Verification items for the finished model (mm, model axes). Face numbers are marked on the shaded views. A direction names the side the tool comes from. Coordinates: 2 decimals unless noted, no trailing zeros. Order: outer loops, then holes, each group sorted by start corner. A loop starts at its lowest first (then second) coordinate and runs counter-clockwise, first axis right, second up. Notation, with made-up numbers: M -13.75,-20.5 L 32.25,-20.5 A20 ccw 32.25,-12.5 Z; hole C -23,75.5 d1. An arc over 180 degrees is marked long. Answer as a JSON object with one key per item and string values. Group by question number.
(1) Cross-section at A-A (x = -34.25). Enter the section's corners in (y, z), plus the area to 3 significant figures.
(2) Cross-section at C-C (z = 10.25). Enter the section's corners in (x, y).
(3) Cross-section at B-B (y = -96). Enter the section's corners in (x, z), plus the area to 3 significant figures.
(4) Cross-section at D-D (x = -40.75). Enter the section's corners in (y, z).
(5) Gauge pin test, flat ends, axial feed: pin 1 Ø1 at (x, z) = (-38, -3.5) entering from -Y; pin 2 Ø6 at (y, z) = (-92, 2) entering from +X (3 decimals); pin 3 Ø1 at (y, z) = (-92, 8) entering from -X. Record the tip position at first contact, or that the pin passes through.
(6) Access from +Z, -Z, +X, -X, +Y, -Y to the whole of each face (thin tool, end or side, straight path). Record for the marked faces 1, 2 and 3.
(7) Material ranges on line 1 (Y direction, x = -36.5, z = -2.5); line 2 (Z direction, x = -35.25, y = -91.5); line 3 (Z direction, x = -39, y = -98), recorded low to high.
from build123d import *

# Parameters (mm, degrees)
SKETCH_1_R      = 5
EXTRUDE_1_DEPTH = 3
SKETCH_2_R      = 3.3
EXTRUDE_2_DEPTH = 12
SKETCH_4_R      = 3.75
EXTRUDE_3_DEPTH = 13


with BuildPart() as part:
    # 草圖1 → 填料-伸長1 (new body)
    with BuildSketch(Plane.XY):
        with Locations((-36.565519845, -95.307444045)):
            Circle(SKETCH_1_R)
    extrude(amount=EXTRUDE_1_DEPTH)

    # 草圖2 → 填料-伸長2 (add)
    with BuildSketch(Plane(origin=(0, 0, 0), x_dir=(-1, 0, 0), z_dir=(0, 0, -1))):
        with Locations((36.565519845, -95.307444045)):
            Circle(SKETCH_2_R)
    extrude(amount=EXTRUDE_2_DEPTH)

    # 草圖4 → 填料-伸長3 (add)
    with BuildSketch(Plane.XY.offset(3)):
        with Locations(Location((-36.565519845, -95.307444045, 0), (0, 0, 180))):
            Circle(SKETCH_4_R)
    extrude(amount=EXTRUDE_3_DEPTH)


solid = part.part
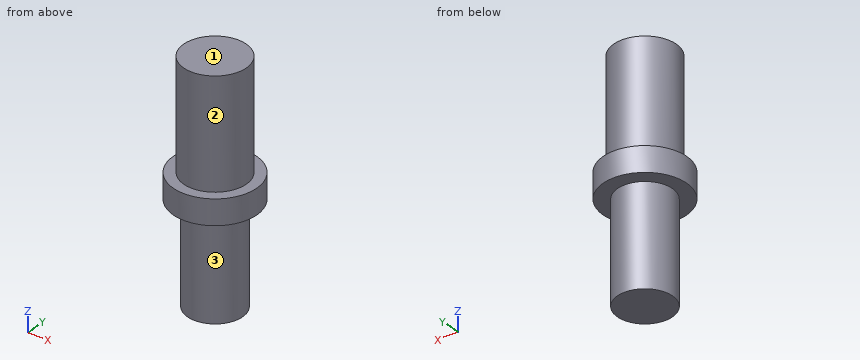
Taken from the geometry:
{
 "1": {"outline": "M -99.74,0 L -97.66,0 L -97.66,-12 L -92.96,-12 L -92.96,0 L -90.88,0 L -90.88,3 L -92.36,3 L -92.36,16 L -98.26,16 L -98.26,3 L -99.74,3 Z", "area": "160 mm²"},
 "2": {"outline": "C -36.57,-95.31 d7.5"},
 "3": {"outline": "M -41.52,0 L -39.79,0 L -39.79,-12 L -33.34,-12 L -33.34,0 L -31.61,0 L -31.61,3 L -32.88,3 L -32.88,16 L -40.25,16 L -40.25,3 L -41.52,3 Z", "area": "203 mm²"},
 "4": {"outline": "M -98.04,0 L -92.57,0 L -92.57,3 L -98.04,3 Z"},
 "5": {"pin 1": "stops at y = -98.47", "pin 2": "stops at x = -31.575", "pin 3": "stops at x = -39.05"},
 "6": {"face 1": "+Z, +X, -X, +Y, -Y", "face 2": "+Z", "face 3": "-Z"},
 "7": {"line 1": "y = -98.61 to -92.01", "line 2": "z = 0 to 3", "line 3": "z = 0 to 16"}
}
